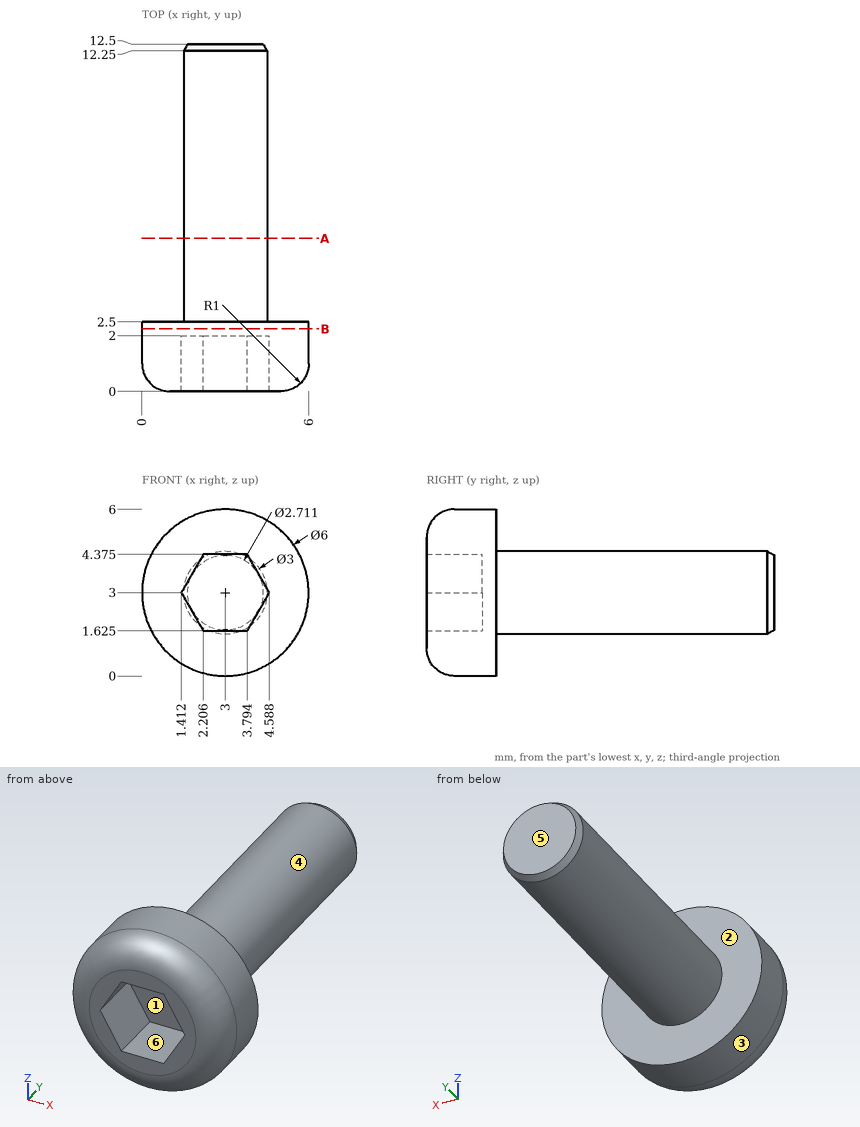
Part print with two shaded views. Sizes in mm from the minimum x, y, z corner. A direction names the side the tool comes from. Round coordinates to 2 decimals unless told otherwise and drop trailing zeros. Write each loop counter-clockwise with the first axis right and the second up, starting at its lowest first coordinate (ties: lowest second). Pieces come first, ordered by that corner, then holes. Notation, with made-up numbers: M -12.5,-13.5 L -1.5,-13.5 A32 cw -1.5,21.5 Z; hole C 52.5,60 d8. An arc over 180 degrees is marked long. Put each result on its own line as item: value. Start each with the question number.
1) Saw through at B-B, the plane y = 2.25. Write the cut outline in (x, z), and give its area (3 significant figures).
2) 3-axis set-ups, long thin cutter, end or side, ignore diameter. For the marked faces 1, 2 and 3: which of +Z, -Z, +X, -X, +Y, -Y reach the whole face in a straight line?
3) Pull direction X, two halves, no side cores. Call the marked faces 4, 5 and 6: pulls with the +X half, pulls with the -X half, needs draft (parallel to the pull), parting line crosses it, or undercut.
4) Pin check, flat tip, straight feed: pin 1 Ø3 at (x, y) = (3.5, 7.5) entering from +Z. Stop position of the tip, or through.
5) Saw through at A-A, the plane y = 5.5. Write the cut outline in (x, z).
6) Drill centre lines: probe 1 along X at (y, z) = (0.5, 1.75) (1 decimal); probe 2 along X at (y, z) = (12, 3); probe 3 along Y at (x, z) = (3.25, 1.85). Where is each one in solid material? Low to high. Write a range as [from, to].
Resolved:
1. outline: C 3,3 d6
1. area: 28.3 mm²
2. face 1: -Y
2. face 2: +Y
2. face 3: +Y, -Y
3. face 4: parting line crosses it
3. face 5: needs draft
3. face 6: undercut
4. pin 1: z = 4.5
5. outline: C 3,3 d3
6. probe 1: [0.4, 2.1], [3.9, 5.6]
6. probe 2: [1.5, 4.5]
6. probe 3: [2, 12.5]
